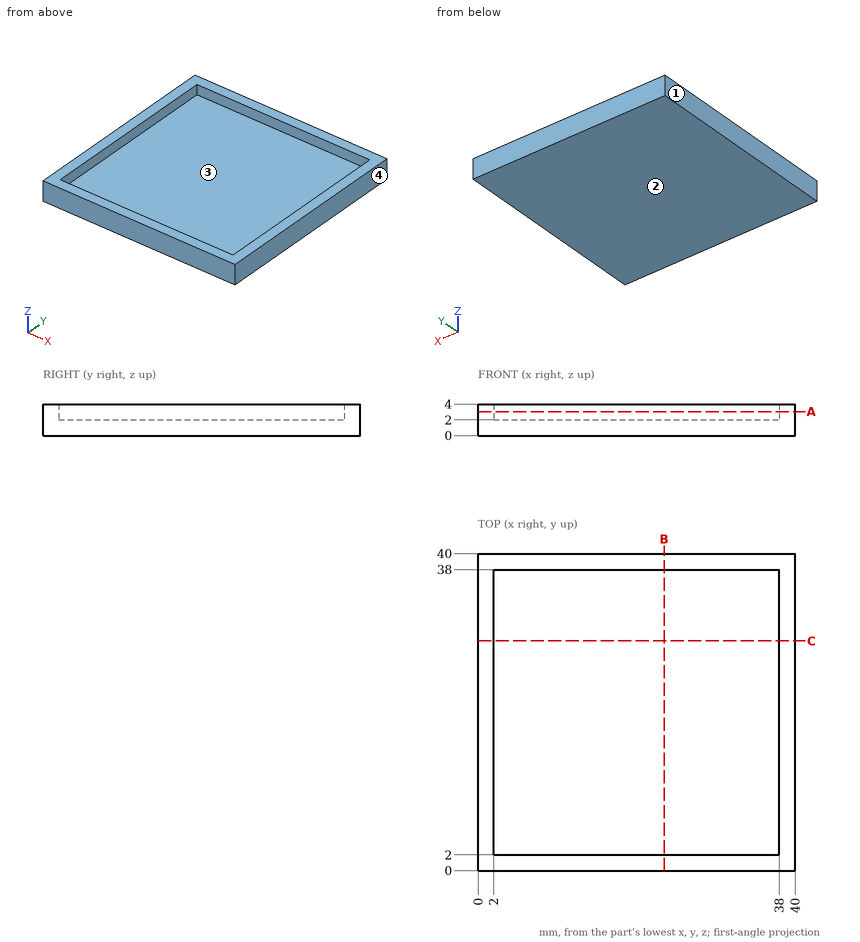
Verification items for this drawing (mm, ordinates from the low corner). Give positions to 0.01 mm unless a question says otherwise; leave off trailing zeros. Loops run counter-clockwise (first coordinate to the right, second up) from the corner with the lowest first, then second, coordinate; pieces in that order, holes last. Notation, with made-up numbers: M 71.5,46 L 90.5,46 A12 ccw 90.5,61 Z; hole C 59,27.25 d4. An arc over 180 degrees is marked long. Answer in a Markdown table with one row per item.
1) Depth check by flat-ended pin: pin 1 (10 mm diameter, centred on x = 31.5, y = 31, fed in from +Z). Enter the tip coordinate at first touch or a pass-through.
Solutions:
| item | result |
|---|---|
| pin 1 | stops at z = 2 |
2) Cross-section at B-B (x = 23.5). Enter the section's corners in (y, z).
Solutions:
| item | result |
|---|---|
| outline | M 0,0 L 40,0 L 40,4 L 38,4 L 38,2 L 2,2 L 2,4 L 0,4 Z |
3) Mould release check, pull along X, two halves, no side actions. Record for the marked faces 1, 2, 3 and 4: released by +X, released by -X, zero draft, split by the parting line, or undercut.
Solutions:
| item | result |
|---|---|
| face 1 | released by -X |
| face 2 | zero draft |
| face 3 | undercut |
| face 4 | released by +X |
4) Thickness scan on line 1 (X direction, y = 34, z = 2.65); line 2 (Z direction, x = 18, y = 10.5). Record the ranges inside material, lowest first.
Solutions:
| item | result |
|---|---|
| line 1 | x = 0 to 2, 38 to 40 |
| line 2 | z = 0 to 2 |
5) Cross-section at A-A (z = 3.05). Enter the section's corners in (x, y), plus the area to 3 significant figures.
Solutions:
| item | result |
|---|---|
| outline | M 0,0 L 40,0 L 40,40 L 0,40 Z; hole M 2,2 L 38,2 L 38,38 L 2,38 Z |
| area | 304 mm^2 |
